```python
from build123d import *

# Parameters (mm, degrees)
F1_DEPTH = 8
F3_DEPTH = 10
F4_R     = 2.75
F5_DEPTH = 25
F6_R     = 4


with BuildPart() as f1:
    # F0 (on Right) → F1 (new body)
    with BuildSketch(Plane.YZ):
        Polygon((0, 26.1), (0, 0), (0, -26.1), (42, -26.1), (42, -46.1), (47, -46.1), (47, -21.1), (9.242641, -21.1), (5, -16.857359), (5, 0), (5, 16.857359), (9.242641, 21.1), (47, 21.1), (47, 46.1), (42, 46.1), (42, 26.1), align=None)
    extrude(amount=F1_DEPTH)

    # F2 (on face) → F3 (join)
    with BuildSketch(Plane.YZ.offset(8)):
        Polygon((5, 13.321825), (12.778175, 21.1), (9.242641, 21.1), (5, 16.857359), align=None)
        Polygon((0, 26.1), (0, -26.1), (42, -26.1), (42, -46.1), (47, -46.1), (47, -21.1), (12.778175, -21.1), (9.242641, -21.1), (5, -16.857359), (5, -13.321825), (5, 0), (5, 13.321825), (5, 16.857359), (9.242641, 21.1), (12.778175, 21.1), (47, 21.1), (47, 46.1), (42, 46.1), (42, 26.1), align=None)
        Polygon((9.242641, -21.1), (12.778175, -21.1), (5, -13.321825), (5, -16.857359), align=None)
    extrude(amount=F3_DEPTH)

    # F4 (on face) → F5 (cut)
    with BuildSketch(Plane.XZ.offset(-42)):
        with Locations((9, 36.1)):
            Circle(F4_R)
        with Locations((9, -36.1)):
            Circle(F4_R)
    extrude(amount=-F5_DEPTH, mode=Mode.SUBTRACT)

    # F6
    f6_edges = [f1.edges().sort_by_distance(p)[0] for p in [
        (9, 0, 26.1),
        (9, 0, -26.1),
        (9, 42, -26.1),
        (9, 42, 26.1),
    ]]
    fillet(f6_edges, radius=F6_R)


solid = f1.part
```
The listing builds one solid part. Answer for the finished solid, in the listing's coordinates (mm). A direction names the side the tool comes from. Coordinates: 2 decimals unless noted, no trailing zeros. Write each loop counter-clockwise with the first axis right and the second up, starting at its lowest first coordinate (ties: lowest second). Pieces come first, ordered by that corner, then holes. Notation, with made-up numbers: (27, -3.75) -> (64, -3.75) arc R9 cw to (64, 11.25) -> close; hole circle Ø3 at (-11, -5). An arc over 180 degrees is marked (long way). Write each question's results on one line, items separated by ' | '. Start each with the question number.
1) A cutting plane is placed at A-A (y = 24). Determine the outline of the cut face in (x, z), then the cut area to 3 significant figures.
2) For a pull along Z with two mould halves and no side action, classify faces 6 (the flat face through (9, 45, 46.1)), 7 (the flat face through (9, 5, 0)), 8 (the flat face through (9, 42, -40)), 9 (the flat face through (8, 8, 18)) as +Z half, -Z half, draft (parallel to the pull), parting line (faces both ways), or undercut.
3) Flat-ended cylindrical pins translate along their axes: pin 1 Ø10 at (x, y) = (9.5, 31.5) entering from -Z; pin 2 Ø9 at (x, y) = (13, 17.5) entering from +Z; pin 3 Ø5.5 at (x, z) = (12, 7.5) entering from +Y; pin 4 Ø5 at (x, z) = (9, -36.1) entering from +Y. Find the tip coordinate at first contact, or state that the pin passes through.
4) Straight lines are drawn through the part: probe 1 along Z at (x, y) = (9, 44.25); probe 2 along Z at (x, y) = (14.5, 17.5); probe 3 along X at (y, z) = (43, -36). For each, find the intervals that lie inside material, in ascending order.
5) A cutting plane is placed at B-B (x = 9). Determine the outline of the cut face in (y, z).
6) A cutting plane is placed at D-D (x = 15). Determine the outline of the cut face in (y, z).
7) A cutting plane is placed at C-C (z = 36.1). Determine the outline of the cut face in (x, y).
8) A tool of negligible diameter and unlimited length cuts with its end or side. For faces 1 (the flat face through (9, 0, 0)), 2 (the flat face through (9, 44, -46.1)), 3 (the flat face through (9, 21, 26.1)), 4 (the flat face through (9, 21, -26.1)), 5 (the flat face through (3.94, 7.09, 18.95)), from which of +Z, -Z, +X, -X, +Y, -Y can it reach the whole face along a straight path? Write none if from no direction.
Values follow:
1) outline: (0, -26.1) -> (18, -26.1) -> (18, -21.1) -> (0, -21.1) -> close; (0, 21.1) -> (18, 21.1) -> (18, 26.1) -> (0, 26.1) -> close | area: 180 mm²
2) face 6: +Z half | face 7: undercut | face 8: draft | face 9: undercut
3) pin 1: z = -26.1 | pin 2: z = 26.1 | pin 3: y = 5 | pin 4: through
4) probe 1: -46.1 to -38.85, -33.35 to -21.1, 21.1 to 33.35, 38.85 to 46.1 | probe 2: -26.1 to -21.1, 21.1 to 26.1 | probe 3: 0 to 6.25, 11.75 to 18
5) outline: (0, -22.1) arc R4 ccw to (4, -26.1) -> (38, -26.1) arc R4 cw to (42, -30.1) -> (42, -33.35) -> (47, -33.35) -> (47, -21.1) -> (12.78, -21.1) -> (5, -13.32) -> (5, 13.32) -> (12.78, 21.1) -> (47, 21.1) -> (47, 33.35) -> (42, 33.35) -> (42, 30.1) arc R4 cw to (38, 26.1) -> (4, 26.1) arc R4 ccw to (0, 22.1) -> close; (42, -46.1) -> (47, -46.1) -> (47, -38.85) -> (42, -38.85) -> close; (42, 38.85) -> (47, 38.85) -> (47, 46.1) -> (42, 46.1) -> close
6) outline: (0, -22.1) arc R4 ccw to (4, -26.1) -> (38, -26.1) arc R4 cw to (42, -30.1) -> (42, -46.1) -> (47, -46.1) -> (47, -21.1) -> (12.78, -21.1) -> (5, -13.32) -> (5, 13.32) -> (12.78, 21.1) -> (47, 21.1) -> (47, 46.1) -> (42, 46.1) -> (42, 30.1) arc R4 cw to (38, 26.1) -> (4, 26.1) arc R4 ccw to (0, 22.1) -> close
7) outline: (0, 42) -> (6.25, 42) -> (6.25, 47) -> (0, 47) -> close; (11.75, 42) -> (18, 42) -> (18, 47) -> (11.75, 47) -> close
8) face 1: +Z, -Z, +X, -X, -Y | face 2: -Z, +X, -X, +Y, -Y | face 3: +Z, +X, -X, -Y | face 4: -Z, +X, -X, -Y | face 5: -X, +Y
